```python
from build123d import *

# Parameters (mm, degrees)
SKETCH1_W                      = 12
SKETCH1_H                      = 8
BOSS_EXTRUDE1_DEPTH            = 700
CBORE_FOR_M3_SHCS1_D           = 3.4
CBORE_FOR_M3_SHCS1_CBORE_D     = 6.5
CBORE_FOR_M3_SHCS1_CBORE_DEPTH = 4.5


with BuildPart() as part:
    # Sketch1 → Boss-Extrude1 (new body)
    with BuildSketch(Plane.XY):
        with Locations((6, 4)):
            Rectangle(SKETCH1_W, SKETCH1_H)
    extrude(amount=BOSS_EXTRUDE1_DEPTH)

    # CBORE for M3 SHCS1 (through all)
    with Locations(Plane(origin=(0, 8, 0), x_dir=(1, 0, 0), z_dir=(0, 1, 0))):
        with Locations((6, -690), (6, -665), (6, -640), (6, -615), (6, -590), (6, -565), (6, -540), (6, -515), (6, -490), (6, -465), (6, -440), (6, -415), (6, -390), (6, -365), (6, -340), (6, -315), (6, -290), (6, -265), (6, -240), (6, -215), (6, -190), (6, -165), (6, -140), (6, -115), (6, -90), (6, -65), (6, -40), (6, -15)):
            CounterBoreHole(CBORE_FOR_M3_SHCS1_D / 2, CBORE_FOR_M3_SHCS1_CBORE_D / 2, CBORE_FOR_M3_SHCS1_CBORE_DEPTH)


solid = part.part
```
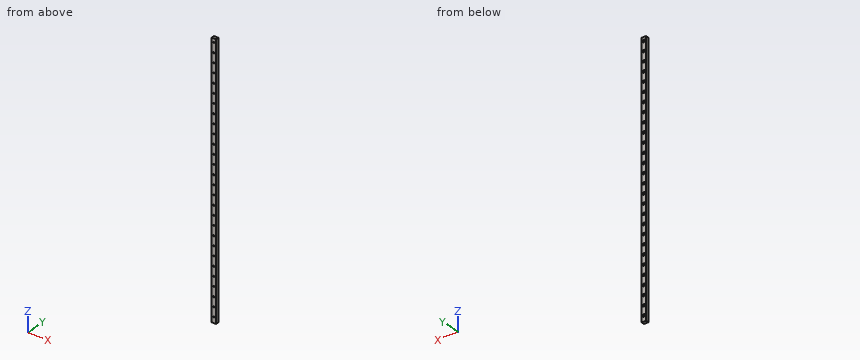
Part model, mm, in its own coordinate system. Coordinates: 2 decimals unless noted, no trailing zeros. Return JSON: item names as keys, results as strings. Group by question number.
Item 1: Cut at A-A (y = 5.25). State how many separate pieces and enclosed holes the cut face has, plus the area to 3 significant figures.
Item 2: Pin check, flat tips, straight feed: pin 1 (4.5 mm diameter, centred on x = 6, z = 215, fed in from +Y); pin 2 (3 mm diameter, centred on x = 6, z = 15, fed in from +Y). Stop position of each tip, or through.
Item 3: Drill centre lines: probe 1 along X at (y, z) = (2.6, 540); probe 2 along X at (y, z) = (4.7, 65); probe 3 along Y at (x, z) = (8, 341.5). Where is each one in solid material? Low to high. Write a range as from..to.
Check values:
{
 "1": {"separate pieces": "1", "enclosed holes": "28", "area": "7,470 mm2"},
 "2": {"pin 1": "stops at y = 3.5", "pin 2": "passes through"},
 "3": {"probe 1": "x = 0..4.3, 7.7..12", "probe 2": "x = 0..2.75, 9.25..12", "probe 3": "y = 0..3.5"}
}
